from build123d import *

# Parameters (mm, degrees)
SKETCH1_W           = 10
SKETCH1_H           = 10
BOSS_EXTRUDE1_DEPTH = 10
SKETCH2_R           = 0.75
CUT_EXTRUDE1_DEPTH  = 170.265249142
SKETCH3_R           = 0.75
CUT_EXTRUDE2_DEPTH  = 170.265249142
CUT_EXTRUDE5_START  = -10
CUT_EXTRUDE5_DEPTH  = 10
SKETCH5_R           = 2.5
CUT_EXTRUDE6_DEPTH  = 170.265249142


with BuildPart() as part:
    # Sketch1 → Boss-Extrude1 (new body)
    with BuildSketch(Plane(origin=(0, 0, 0), x_dir=(0, 0, -1), z_dir=(1, 0, 0))):
        with BuildLine():
            Line((0, 109.22405545), (0, -43.10336506))
            ThreePointArc((0, -43.10336506), (0.541577594, -48.278843147), (2.142845875, -53.230087397))
            ThreePointArc((2.142845875, -53.230087397), (-15.125529103, -79.668997921), (-32.212650318, -53.112585274))
            ThreePointArc((-32.212650318, -53.112585274), (-30.559421631, -48.088849966), (-30, -42.82975033))
            Line((-30, -42.82975033), (-30, 109.060958061))
            ThreePointArc((-30, 109.060958061), (-31.291322972, 116.99182394), (-35.031890687, 124.103385075))
            ThreePointArc((-35.031890687, 124.103385075), (-15.112146754, 164.150992221), (4.970722417, 124.184939097))
            ThreePointArc((4.970722417, 124.184939097), (1.275203483, 117.106569656), (0, 109.22405545))
        make_face()
        with Locations((-15.061172266, 83.959086258)):
            Rectangle(SKETCH1_W, SKETCH1_H, mode=Mode.SUBTRACT)
        with Locations((-15.061172266, -26.040913742)):
            Rectangle(SKETCH1_W, SKETCH1_H, mode=Mode.SUBTRACT)
    extrude(amount=BOSS_EXTRUDE1_DEPTH)

    # Sketch2 → Cut-Extrude1 (cut, through all)
    with BuildSketch(Plane(origin=(10, 0, 0), x_dir=(0, 0, -1), z_dir=(1, 0, 0))):
        with Locations((-15.061172266, 143.397777589)):
            Circle(SKETCH2_R)
        with Locations((-19.311172266, 139.147777589)):
            Circle(SKETCH2_R)
        with Locations((-10.811172266, 139.147777589)):
            Circle(SKETCH2_R)
        with Locations((-15.061172266, 134.897777589)):
            Circle(SKETCH2_R)
    extrude(amount=-CUT_EXTRUDE1_DEPTH, mode=Mode.SUBTRACT)

    # Sketch3 → Cut-Extrude2 (cut, through all)
    with BuildSketch(Plane(origin=(10, 0, 0), x_dir=(0, 0, -1), z_dir=(1, 0, 0))):
        with Locations((-19.311172266, -69.352222411)):
            Circle(SKETCH3_R)
        with Locations((-15.061172266, -65.102222411)):
            Circle(SKETCH3_R)
        with Locations((-10.811172266, -69.352222411)):
            Circle(SKETCH3_R)
        with Locations((-15.061172266, -73.602222411)):
            Circle(SKETCH3_R)
    extrude(amount=-CUT_EXTRUDE2_DEPTH, mode=Mode.SUBTRACT)

    # Sketch4 → Cut-Extrude5 (cut)
    with BuildSketch(Plane(origin=(10, 0, 0), x_dir=(0, 0, -1), z_dir=(1, 0, 0)).offset(CUT_EXTRUDE5_START)):
        with BuildLine():
            Line((-30, -42.82975033), (-30, -33.739733883))
            Line((-30, -33.739733883), (-50.712575643, -33.739733883))
            Line((-50.712575643, -33.739733883), (-50.712575643, -86.676053834))
            Line((-50.712575643, -86.676053834), (22.03762198, -86.676053834))
            Line((22.03762198, -86.676053834), (22.03762198, -33.739733883))
            Line((22.03762198, -33.739733883), (0, -33.739733883))
            Line((0, -33.739733883), (0, -43.10336506))
            ThreePointArc((0, -43.10336506), (0.541577594, -48.278843147), (2.142845875, -53.230087397))
            ThreePointArc((2.142845875, -53.230087397), (-15.125529103, -79.668997921), (-32.212650318, -53.112585274))
            ThreePointArc((-32.212650318, -53.112585274), (-30.559421631, -48.088849966), (-30, -42.82975033))
        make_face()
        with BuildLine():
            Line((-30, -46.956071773), (-30, -42.82975033))
            ThreePointArc((-30, -42.82975033), (-30.559421631, -48.088849966), (-32.212650318, -53.112585274))
            ThreePointArc((-32.212650318, -53.112585274), (-15.125529103, -79.668997921), (2.142845875, -53.230087397))
            ThreePointArc((2.142845875, -53.230087397), (0.541577594, -48.278843147), (0, -43.10336506))
            Line((0, -43.10336506), (0, -33.739733883))
            Line((0, -33.739733883), (-0.122344533, -33.739733883))
            Line((-0.122344533, -33.739733883), (-0.122344533, -46.956071773))
            ThreePointArc((-0.122344533, -46.956071773), (-1.211385526, -52.547049066), (-4.319271357, -57.320526105))
            ThreePointArc((-4.319271357, -57.320526105), (-7.279094989, -62.31182931), (-7.666142531, -68.101808395))
            ThreePointArc((-7.666142531, -68.101808395), (-15.061172266, -76.852222411), (-22.456202002, -68.101808395))
            ThreePointArc((-22.456202002, -68.101808395), (-22.843249544, -62.31182931), (-25.803073176, -57.320526105))
            ThreePointArc((-25.803073176, -57.320526105), (-28.910959007, -52.547049066), (-30, -46.956071773))
        make_face()
    extrude(amount=CUT_EXTRUDE5_DEPTH, mode=Mode.SUBTRACT)

    # Sketch5 → Cut-Extrude6 (cut, through all)
    with BuildSketch(Plane(origin=(10, 0, 0), x_dir=(0, 0, -1), z_dir=(1, 0, 0))):
        with Locations((-15.061172266, 139.147777589)):
            Circle(SKETCH5_R)
    extrude(amount=-CUT_EXTRUDE6_DEPTH, mode=Mode.SUBTRACT)


solid = part.part
Design review of the part built by this model. Coordinates are the model's own, in mm. A direction names the side the tool comes from. Round coordinates to 2 decimals unless told otherwise and drop trailing zeros. Write each loop counter-clockwise with the first axis right and the second up, starting at its lowest first coordinate (ties: lowest second). Pieces come first, ordered by that corner, then holes. Notation, with made-up numbers: (26.5, 84) -> (30.5, 84) arc R33 ccw to (30.5, 121) -> close; hole circle Ø4 at (-16.75, -39.5). An arc over 180 degrees is marked (long way). One line per question, with ' | ' between items.
(1) Take a section at B-B, the plane y = 16.5. State the section outline as (x, z) points.
Result sheet:
outline: (0, 0) -> (10, 0) -> (10, 30) -> (0, 30) -> close
(2) Draft analysis for pull direction Z (two halves, no side actions). For faces 4 (the flat face through (5, -21.041, 15)), 5 (the flat face through (5, 30, 30)), 6 (the cylindrical face through (4.93, -76.85, 14.88)), state which applies: released by +Z, released by -Z, zero draft, split by the parting line, or undercut.
Result sheet:
face 4: undercut | face 5: released by +Z | face 6: split by the parting line
(3) Wall thickness on line 1 (Z direction, x = 1.75, y = 72); line 2 (Y direction, x = 9.25, z = 11); line 3 (Z direction, x = 2, y = 143.5): over which ranges is each line inside the solid? List them lowest first. Write a range as [from, to].
Result sheet:
line 1: [0, 30] | line 2: [-75.66, -70.08], [-68.63, -31.04], [-21.04, 78.96], [88.96, 138.42], [139.87, 163.82] | line 3: [-9.56, 14.32], [15.8, 39.68]
(4) Take a section at A-A, the plane x = 7.25. State how many separate pieces and enclosed holes the cut face has, and give its area (3 significant figures).
Result sheet:
separate pieces: 1 | enclosed holes: 11 | area: 7,190 mm2
(5) Take a section at C-C, the plane y = -36.5. State the section outline as (x, z) points, and give its area (3 significant figures).
Result sheet:
outline: (0, 0.12) -> (10, 0.12) -> (10, 30) -> (0, 30) -> close | area: 299 mm2
(6) Insertion check: P1, Ø1.7, axis at y = -69.35, z = 10.81, coming from the -X side; P2, Ø1, axis at x = 5, y = 86, coming from the +Z side; P3, Ø5, axis at x = 8, y = 75.5, coming from the -Z side. Each pin has a flat end and moves straight along its axis. Give the tip position at first contact, or say it passes through.
Result sheet:
P1: x = 0 | P2: z = 30 | P3: z = 0
(7) Machinability: for faces 1 (the flat face through (5, -40, 0.122)), 2 (the flat face through (5, 84, 10.061)), 3 (the cylindrical face through (4.93, -52.62, 28.88)), which of the approach directions +Z, -Z, +X, -X, +Y, -Y give a long, thin tool a straight path to every point of the face, cutting with its end or side? Answer none if there is none.
Result sheet:
face 1: -Z, +X, -X, -Y | face 2: +X, -X | face 3: +Z, +X, -X, -Y
